Can you work these out from the model? Positions are in its coordinate system, mm. Face numbers are marked on the shaded views. A direction names the side the tool comes from. Round coordinates to 2 decimals unless told otherwise and drop trailing zeros. Loops run counter-clockwise (first coordinate to the right, second up) from the corner with the lowest first, then second, coordinate; pieces in that order, holes last. Notation, with made-up numbers: M -5,7 L -1,7 A24 ccw -1,43 Z; hole C 11.25,-16 d10. An arc over 180 degrees is marked long. Use a Markdown table: item, result. Add a question column.
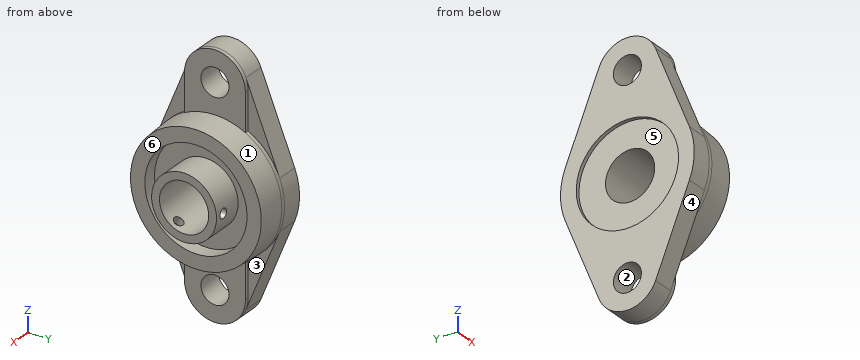
```python
from build123d import *

# Parameters (mm, degrees)
EXTRUDE_1_DEPTH               = 2
EXTRUDE_2_DEPTH               = 11
SKETCH_3_R                    = 34
EXTRUDE_3_DEPTH               = 14
EXTRUDE_3_TAPER               = 3
HOLE_WIZARD_M45_1_D           = 52
HOLE_WIZARD_M45_1_DEPTH       = 7.15
SKETCH_6_W                    = 15.85
SKETCH_6_H                    = 16.5
HOLE_WIZARD_14_25_14_25_1_D   = 14.25
HOLE_WIZARD_M24_1_D           = 25
HOLE_WIZARD_M24_1_DEPTH       = 35.7
HOLE_WIZARD_M24_1_CBORE_D     = 52
HOLE_WIZARD_M24_1_CBORE_DEPTH = 2
SKETCH_11_W                   = 2.4585
SKETCH_11_H                   = 61.03580457
HOLE_WIZARD_2_D               = 4.917
HOLE_WIZARD_2_DEPTH           = 21.744153324


with BuildPart() as part:
    # 草图1 → 凸台-拉伸1 (new body)
    with BuildSketch(Plane(origin=(13, 0, 0), x_dir=(0, 0, -1), z_dir=(1, 0, 0))):
        with BuildLine():
            Line((49.5, 15.5), (30.261361503, 15.5))
            ThreePointArc((30.261361503, 15.5), (0, 34), (-30.261361503, 15.5))
            Line((-30.261361503, 15.5), (-49.5, 15.5))
            ThreePointArc((-49.5, 15.5), (-65, 0), (-49.5, -15.5))
            Line((-49.5, -15.5), (-30.261361503, -15.5))
            ThreePointArc((-30.261361503, -15.5), (0, -34), (30.261361503, -15.5))
            Line((30.261361503, -15.5), (49.5, -15.5))
            ThreePointArc((49.5, -15.5), (65, 0), (49.5, 15.5))
        make_face()
    extrude(amount=-EXTRUDE_1_DEPTH)

    # 草图2 → 凸台-拉伸2 (add)
    with BuildSketch(Plane.ZY.offset(-11)):
        with BuildLine():
            Line((12.707070707, 31.536175324), (55.292929293, 14.376785809))
            ThreePointArc((55.292929293, 14.376785809), (65, 0), (55.292929293, -14.376785809))
            Line((55.292929293, -14.376785809), (12.707070707, -31.536175324))
            ThreePointArc((12.707070707, -31.536175324), (0, -34), (-12.707070707, -31.536175324))
            Line((-12.707070707, -31.536175324), (-55.292929293, -14.376785809))
            ThreePointArc((-55.292929293, -14.376785809), (-65, 0), (-55.292929293, 14.376785809))
            Line((-55.292929293, 14.376785809), (-12.707070707, 31.536175324))
            ThreePointArc((-12.707070707, 31.536175324), (0, 34), (12.707070707, 31.536175324))
        make_face()
    extrude(amount=EXTRUDE_2_DEPTH)

    # 草图3 → 凸台-拉伸3 (add)
    with BuildSketch(Plane(origin=(13, 0, 0), x_dir=(0, 0, -1), z_dir=(1, 0, 0))):
        Circle(SKETCH_3_R)
    extrude(amount=EXTRUDE_3_DEPTH, taper=EXTRUDE_3_TAPER)

    # M45 间隙孔1
    with Locations(Plane(origin=(27, 0, 0), x_dir=(0, 0, -1), z_dir=(1, 0, 0))):
        with Locations((0, 0)):
            Hole(HOLE_WIZARD_M45_1_D / 2, depth=HOLE_WIZARD_M45_1_DEPTH)

    # 草图6 → 旋转1 (revolve)
    with BuildSketch(Plane(origin=(0, 0, 0), x_dir=(-1, 0, 0), z_dir=(0, 0, -1))):
        with Locations((-27.775, 8.25)):
            Rectangle(SKETCH_6_W, SKETCH_6_H)
    revolve(axis=Axis((35.7, 0, 0), (-1, 0, 0)))

    # Ø14.25 (14.25) 直径孔1 (through all)
    with Locations(Plane(origin=(13, 0, 0), x_dir=(0, 0, -1), z_dir=(1, 0, 0))):
        with Locations((-49.5, 0), (49.5, 0)):
            Hole(HOLE_WIZARD_14_25_14_25_1_D / 2)

    # M24 六角头螺栓的柱形沉头孔1
    with Locations(Plane.ZY):
        with Locations((0, 0)):
            CounterBoreHole(HOLE_WIZARD_M24_1_D / 2, HOLE_WIZARD_M24_1_CBORE_D / 2, HOLE_WIZARD_M24_1_CBORE_DEPTH, depth=HOLE_WIZARD_M24_1_DEPTH)

    # 草图11 → 孔1 (revolve, cut)
    with BuildSketch(Plane(origin=(30.7, -6.127923338, -10.613874566), x_dir=(0, -0.866025404, 0.5), z_dir=(1, 0, 0))):
        with Locations((1.22925, 30.517902285)):
            Rectangle(SKETCH_11_W, SKETCH_11_H)
    revolve(axis=Axis((30.7, -61.127923338, -105.876668983), (0, 0.5, 0.866025404)), mode=Mode.SUBTRACT)

    # 孔2
    with Locations(Plane(origin=(0, 12.255846676, 0), x_dir=(-1, 0, 0), z_dir=(0, -1, 0))):
        with Locations((-30.7, 0)):
            Hole(HOLE_WIZARD_2_D / 2, depth=HOLE_WIZARD_2_DEPTH)


solid = part.part
```
(1) Suppose I cut it at D-D on z = -53. List the corners of the cut face in (x, y) for me, and give its area (3 significant figures).
(2) Suppose I cut it at B-B on x = 30.7. List the corners of the cut face in (y, z) for me.
(3) Suppose I cut it at A-A on z = 0. List the corners of the cut face in (x, y) for me, and give its area (3 significant figures).
(4) Suppose I cut it at C-C on y = 0. Count the separate pieces of the cut face and the enclosed holes in it, and give its area (3 significant figures).
(5) On a 3-axis mill with a long thin cutter (end or side, diameter ignored), from which of +Z, -Z, +X, -X, +Y, -Y can I reach the whole of each face in a straight line? I mean the marked faces 4, 5 and 6. Say none if no direction works.
(6) If I drill on probe 1 along Y at (x, z) = (28, 0); probe 2 along X at (y, z) = (-21, 12.5); probe 3 along X at (y, z) = (3, 41), over which ranges is the centre line in solid material (lowest first)? Write a range as [from, to].
(7) Thinking about a two-plate mould opening in Z: for the marked faces 1, 2 and 3, which applies, released by +Z, released by -Z, zero draft, split by the parting line, or undercut?
(8) I'm going to push flat-ended pins straight in: pin 1 (0.6 mm diameter, centred on x = 12, z = -38.5, fed in from -Y); pin 2 (12 mm diameter, centred on x = 11.5, y = -7, fed in from +Z); pin 3 (12 mm diameter, centred on x = 26, y = 13, fed in from +Z); pin 4 (1.5 mm diameter, centred on x = 28, z = -22.5, fed in from +Y). Where does each tip first touch, or does it pass through?
Results below:
| question | item | result |
|---|---|---|
| 1 | outline | M 0,-15.3 L 11,-15.3 L 11,-15.1 L 13,-15.1 L 13,-6.21 L 0,-6.21 Z; M 0,6.21 L 13,6.21 L 13,15.1 L 11,15.1 L 11,15.3 L 0,15.3 Z |
| 1 | area | 236 mm² |
| 2 | outline | M -10.29,-12.9 L -8.26,-9.38 A12.5 cw long 12.26,2.46 L 16.32,2.46 A16.5 ccw long Z; M -6.03,-15.36 A16.5 ccw 16.32,-2.46 L 12.26,-2.46 A12.5 cw -4,-11.84 Z |
| 3 | outline | M 0,-34 L 13,-34 L 27,-33.27 L 27,-26 L 19.85,-26 L 19.85,-16.5 L 35.7,-16.5 L 35.7,-12.5 L 2,-12.5 L 2,-26 L 0,-26 Z; M 0,26 L 2,26 L 2,12.5 L 28.24,12.5 L 28.24,16.5 L 19.85,16.5 L 19.85,26 L 27,26 L 27,33.27 L 13,34 L 0,34 Z; M 33.16,12.5 L 35.7,12.5 L 35.7,16.5 L 33.16,16.5 Z |
| 3 | area | 1,010 mm² |
| 4 | separate pieces | 4 |
| 4 | enclosed holes | 0 |
| 4 | area | 1,470 mm² |
| 5 | face 4 | -Z, +X, -X, -Y |
| 5 | face 5 | -X |
| 5 | face 6 | +X |
| 6 | probe 1 | y = [-16.5, -12.5], [12.5, 16.5] |
| 6 | probe 2 | x = [2, 19.85] |
| 6 | probe 3 | x = [0, 13] |
| 7 | face 1 | split by the parting line |
| 7 | face 2 | undercut |
| 7 | face 3 | zero draft |
| 8 | pin 1 | stops at y = -15.5 |
| 8 | pin 2 | stops at z = 64.97 |
| 8 | pin 3 | stops at z = 32.61 |
| 8 | pin 4 | passes through |
